Work out the finished part from the listing and answer in its coordinate system (mm). A direction names the side the tool comes from. Give positions to 0.01 mm unless a question says otherwise; leave off trailing zeros. Order: outer loops, then holes, each group sorted by start corner. A loop starts at its lowest first (then second) coordinate and runs counter-clockwise, first axis right, second up.
```python
from build123d import *

# Parameters (mm, degrees)
EXTRUDE_1_DEPTH     = 4
SKETCH_5_R          = 1.65
CUT_EXTRUDE_1_DEPTH = 2.1


with BuildPart() as part:
    # Sketch 1 → Extrude 1 (new body)
    with BuildSketch(Plane(origin=(0, 0, 0), x_dir=(1, 0, 0), z_dir=(0, 1, 0))):
        with BuildLine():
            Line((85.982202548, 23.730183562), (80.444848449, 19.403928396))
            ThreePointArc((80.444848449, 19.403928396), (78.581927501, 18.960188067), (77.028827056, 20.08057146))
            Line((77.028827056, 20.08057146), (77.028827056, 67.115745446))
            Line((77.028827056, 67.115745446), (-87.971172944, 67.115745446))
            ThreePointArc((-87.971172944, 67.115745446), (-98.577774662, 62.722347164), (-102.971172944, 52.115745446))
            Line((-102.971172944, 52.115745446), (-102.971172944, -47.884254554))
            ThreePointArc((-102.971172944, -47.884254554), (-98.577774662, -58.490856271), (-87.971172944, -62.884254554))
            Line((-87.971172944, -62.884254554), (77.028827056, -62.884254554))
            Line((77.028827056, -62.884254554), (77.028827056, -15.849080568))
            ThreePointArc((77.028827056, -15.849080568), (78.581927501, -14.728697175), (80.444848449, -15.172437504))
            Line((80.444848449, -15.172437504), (85.982202548, -19.49869267))
            ThreePointArc((85.982202548, -19.49869267), (87.774058006, -19.687024267), (88.728827056, -18.159074389))
            Line((88.728827056, -18.159074389), (88.728827056, 22.390565281))
            ThreePointArc((88.728827056, 22.390565281), (87.774058006, 23.91851516), (85.982202548, 23.730183562))
        make_face()
    extrude(amount=EXTRUDE_1_DEPTH)

    # Sketch 5 → Cut-Extrude 1 (cut)
    with BuildSketch(Plane(origin=(0, 4, 0), x_dir=(1, 0, 0), z_dir=(0, 1, 0))):
        with Locations(Location((84.828827056, -13.648405937, 0), (0, 0, 270))):
            Circle(SKETCH_5_R)
        with Locations(Location((84.828827056, 2.115745446, 0), (0, 0, 270))):
            Circle(SKETCH_5_R)
        with Locations(Location((84.828827056, 17.87989683, 0), (0, 0, 270))):
            Circle(SKETCH_5_R)
        with Locations(Location((71.11417076, 62.115745446, 0), (0, 0, 270))):
            Circle(SKETCH_5_R)
        with Locations(Location((52.11417076, 62.115745446, 0), (0, 0, 270))):
            Circle(SKETCH_5_R)
        with Locations(Location((33.11417076, 62.115745446, 0), (0, 0, 270))):
            Circle(SKETCH_5_R)
        with Locations(Location((14.11417076, 62.115745446, 0), (0, 0, 270))):
            Circle(SKETCH_5_R)
        with Locations(Location((-4.88582924, 62.115745446, 0), (0, 0, 270))):
            Circle(SKETCH_5_R)
        with Locations(Location((-23.88582924, 62.115745446, 0), (0, 0, 270))):
            Circle(SKETCH_5_R)
        with Locations(Location((-42.88582924, 62.115745446, 0), (0, 0, 270))):
            Circle(SKETCH_5_R)
        with Locations(Location((-61.88582924, 62.115745446, 0), (0, 0, 270))):
            Circle(SKETCH_5_R)
        with Locations(Location((-80.88582924, 62.115745446, 0), (0, 0, 270))):
            Circle(SKETCH_5_R)
        with Locations(Location((-94.335133975, 58.479706477, 0), (0, 0, 270))):
            Circle(SKETCH_5_R)
        with Locations(Location((-97.971172944, 44.88442265, 0), (0, 0, 270))):
            Circle(SKETCH_5_R)
        with Locations(Location((-97.971172944, 27.74775595, 0), (0, 0, 270))):
            Circle(SKETCH_5_R)
        with Locations(Location((-97.971172944, 10.61108925, 0), (0, 0, 270))):
            Circle(SKETCH_5_R)
        with Locations(Location((-97.971172944, -6.52557745, 0), (0, 0, 270))):
            Circle(SKETCH_5_R)
        with Locations(Location((-97.971172944, -23.66224415, 0), (0, 0, 270))):
            Circle(SKETCH_5_R)
        with Locations(Location((-97.971172944, -40.79891085, 0), (0, 0, 270))):
            Circle(SKETCH_5_R)
        with Locations(Location((-94.335133975, -54.248215584, 0), (0, 0, 270))):
            Circle(SKETCH_5_R)
        with Locations(Location((-80.88582924, -57.884254554, 0), (0, 0, 270))):
            Circle(SKETCH_5_R)
        with Locations(Location((-61.88582924, -57.884254554, 0), (0, 0, 270))):
            Circle(SKETCH_5_R)
        with Locations(Location((-42.88582924, -57.884254554, 0), (0, 0, 270))):
            Circle(SKETCH_5_R)
        with Locations(Location((-23.88582924, -57.884254554, 0), (0, 0, 270))):
            Circle(SKETCH_5_R)
        with Locations(Location((-4.88582924, -57.884254554, 0), (0, 0, 270))):
            Circle(SKETCH_5_R)
        with Locations(Location((14.11417076, -57.884254554, 0), (0, 0, 270))):
            Circle(SKETCH_5_R)
        with Locations(Location((33.11417076, -57.884254554, 0), (0, 0, 270))):
            Circle(SKETCH_5_R)
        with Locations(Location((52.11417076, -57.884254554, 0), (0, 0, 270))):
            Circle(SKETCH_5_R)
        with Locations(Location((71.11417076, -57.884254554, 0), (0, 0, 270))):
            Circle(SKETCH_5_R)
    extrude(amount=-CUT_EXTRUDE_1_DEPTH, mode=Mode.SUBTRACT)


solid = part.part
```
1. Which of the six approach directions +Z, -Z, +X, -X, +Y, -Y give full straight-line access (tool end or side, diameter ignored) to faces 4 (the face through (-98.694, 1.972, 58.374)), 5 (the face through (83.252, 1.972, -21.597))?
Findings below:
face 4: +Z, -X, +Y, -Y
face 5: -Z, +Y, -Y
2. Given P1, Ø12, axis at x = 41, z = -21, coming from the -Y side; P2, Ø2, axis at x = -97.97, z = -44.88, coming from the +Y side, each flat-ended and moving along its own axis, determine where each tip first touches the part or whether it passes through.
Findings below:
P1: stops at y = 0
P2: stops at y = 1.9
3. The part is cut by section A-A (y = 0.8). Write down the section's boundary in (x, z).
Findings below:
outline: (-102.97, -52.12) arc R15 ccw to (-87.97, -67.12) - (77.03, -67.12) - (77.03, -20.08) arc R2.3 cw to (80.44, -19.4) - (85.98, -23.73) arc R1.7 ccw to (88.73, -22.39) - (88.73, 18.16) arc R1.7 ccw to (85.98, 19.5) - (80.44, 15.17) arc R2.3 cw to (77.03, 15.85) - (77.03, 62.88) - (-87.97, 62.88) arc R15 ccw to (-102.97, 47.88) - close
4. The mould has two halves that part along X. Classify faces 1 (the face through (-4, 2, -67.116)), 2 (the face through (83.175, 1.972, 17.305)), 3 (the face through (-102.971, 2, -3)): pulls with the +X half, pulls with the -X half, needs draft (parallel to the pull), parting line crosses it, or undercut.
Findings below:
face 1: needs draft
face 2: undercut
face 3: pulls with the -X half
5. Straight lines are drawn through the part: probe 1 along Z at (x, y) = (-62, 2.4); probe 2 along X at (y, z) = (3.65, -18); probe 3 along X at (y, z) = (2.7, -25.5). For each, find the intervals that lie inside material, in ascending order.
Findings below:
probe 1: z = -67.12 to -63.76, -60.47 to 56.24, 59.53 to 62.88
probe 2: x = -102.97 to 83.18, 86.47 to 88.73
probe 3: x = -102.97 to 77.03
